Study the drawing (mm; zero at the part's minimum x, y, z) and answer. A direction names the side the tool comes from. Coordinates: 2 decimals unless noted, no trailing zeros. Loops run counter-clockwise (first coordinate to the right, second up) from the corner with the lowest first, then second, coordinate; pieces in that order, holes last. Notation, with made-up numbers: (11.5, 31.25) - (37.5, 31.25) arc R23 ccw to (37.5, 59.25) - close; hole circle Ø9 at (27, 20). An arc over 180 degrees is marked (long way). One line per item, written item: value. Start each with the question number.
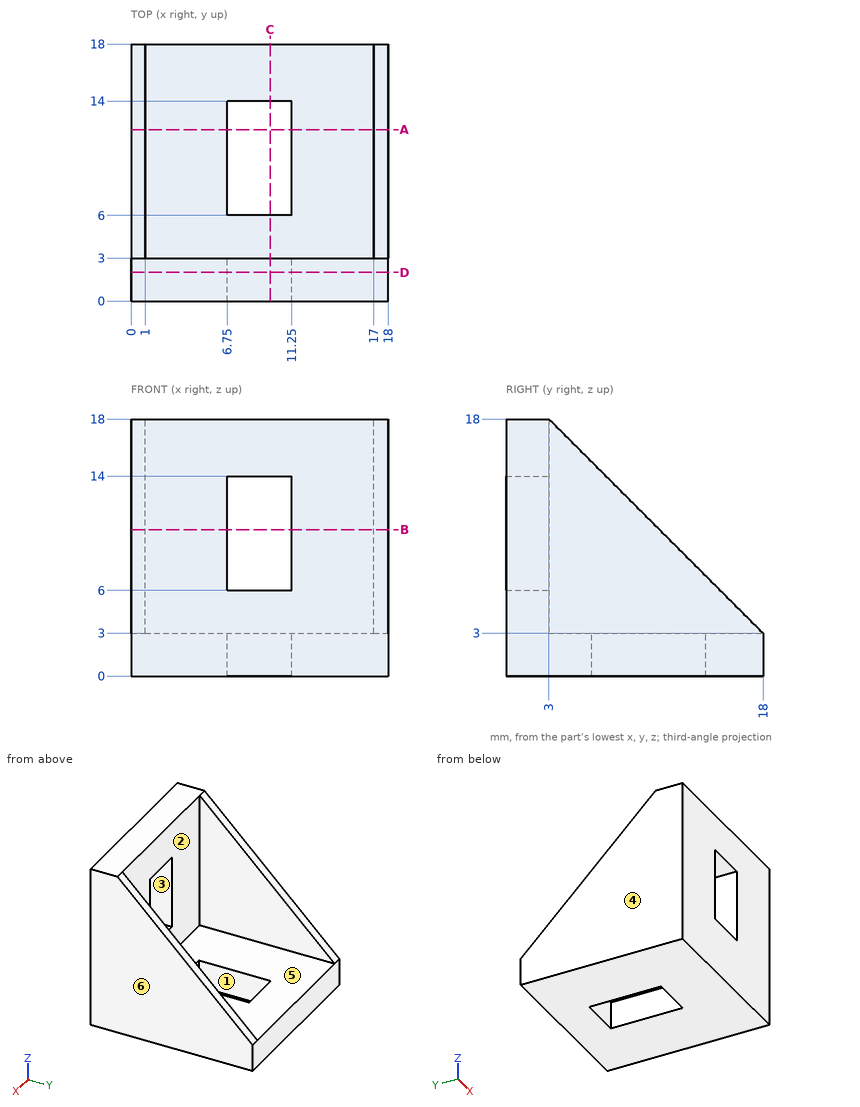
1) Section D-D, the plane y = 2 is taken. Determine the outline of the cut face in (x, z).
2) Section C-C, the plane x = 9.75 is taken. Determine the outline of the cut face in (y, z), and give its area (3 significant figures).
3) Straight lines are drawn through the part: L1, parallel to X at y = 7, z = 5.5; L2, parallel to X at y = 13, z = 2.75; L3, parallel to Z at x = 10.5, y = 2. For each, find the intervals that lie inside material, in ascending order.
4) For the marked faces 1, 2 and 3, determine the directions among +Z, -Z, +X, -X, +Y, -Y from which every point of the face is accessible in a straight line to the end or side of a thin tool.
5) Section A-A, the plane y = 12 is taken. Determine the outline of the cut face in (x, z), and give its area (3 significant figures).
6) Flat-ended cylindrical pins translate along their axes: P1, Ø4, axis at x = 5.5, y = 10, coming from the +Z side; P2, Ø7.5, axis at x = 7, z = 11.5, coming from the +Y side. Find the tip coordinate at first contact, or state that the pin passes through.
7) Determine the mould class of the marked faces 4, 5 and 6 for opening direction X: released by +X, released by -X, zero draft, split by the parting line, or undercut.
8) Section B-B, the plane z = 10.25 is taken. Determine the outline of the cut face in (x, y), and give its area (3 significant figures).
Answer below:
1. outline: (0, 0) - (18, 0) - (18, 18) - (0, 18) - close; hole (6.75, 6) - (11.25, 6) - (11.25, 14) - (6.75, 14) - close
2. outline: (0, 0) - (6, 0) - (6, 3) - (3, 3) - (3, 6) - (0, 6) - close; (0, 14) - (3, 14) - (3, 18) - (0, 18) - close; (14, 0) - (18, 0) - (18, 3) - (14, 3) - close
2. area: 51.0 mm2
3. L1: 0 to 1, 17 to 18
3. L2: 0 to 6.75, 11.25 to 18
3. L3: 0 to 6, 14 to 18
4. face 1: +Z, -Z
4. face 2: +Z, +Y
4. face 3: +Y, -Y
5. outline: (0, 0) - (6.75, 0) - (6.75, 3) - (1, 3) - (1, 9) - (0, 9) - close; (11.25, 0) - (18, 0) - (18, 9) - (17, 9) - (17, 3) - (11.25, 3) - close
5. area: 52.5 mm2
6. P1: z = 3
6. P2: y = 3
7. face 4: released by -X
7. face 5: undercut
7. face 6: released by +X
8. outline: (0, 0) - (6.75, 0) - (6.75, 3) - (1, 3) - (1, 10.75) - (0, 10.75) - close; (11.25, 0) - (18, 0) - (18, 10.75) - (17, 10.75) - (17, 3) - (11.25, 3) - close
8. area: 56.0 mm2
